```python
from build123d import *

# Parameters (mm, degrees)
BOSS_EXTRUDE1_DEPTH      = 20
SCHIZZO6_R               = 3
TAGLIO_ESTRUSIONE1_DEPTH = 282.870567709


with BuildPart() as part:
    # Sketch1 → Boss-Extrude1 (new body)
    with BuildSketch(Plane.XY):
        Polygon((35, -64), (-43.999999997, -64), (-43.999999997, 126), (35, 126), (251.346408251, 59.694869443), (251.346408251, -64), align=None)
    extrude(amount=BOSS_EXTRUDE1_DEPTH)

    # Schizzo6 → Taglio-Estrusione1 (cut, through all)
    with BuildSketch(Plane.XY.offset(20)):
        with Locations((28.5, -53.5)):
            Circle(SCHIZZO6_R)
        with Locations((-28.5, -53.5)):
            Circle(SCHIZZO6_R)
        with Locations((-28.5, -8.5)):
            Circle(SCHIZZO6_R)
        with Locations((28.5, -8.5)):
            Circle(SCHIZZO6_R)
        with Locations((28.5, 115.5)):
            Circle(SCHIZZO6_R)
        with Locations((28.5, 70.5)):
            Circle(SCHIZZO6_R)
        with Locations((-28.5, 115.5)):
            Circle(SCHIZZO6_R)
        with Locations((-28.5, 70.5)):
            Circle(SCHIZZO6_R)
        with Locations((-38.999999997, 20.3)):
            Circle(SCHIZZO6_R)
        with Locations((-38.999999997, 42.3)):
            Circle(SCHIZZO6_R)
        with Locations((-0.999999997, 20.3)):
            Circle(SCHIZZO6_R)
        with Locations((-0.999999997, 42.3)):
            Circle(SCHIZZO6_R)
    extrude(amount=-TAGLIO_ESTRUSIONE1_DEPTH, mode=Mode.SUBTRACT)


solid = part.part
```
Input: part model. Units: mm. Frame: model coordinates. Round coordinates to 2 decimals unless told otherwise and drop trailing zeros. Order: outer loops, then holes, each group sorted by start corner. A loop starts at its lowest first (then second) coordinate and runs counter-clockwise, first axis right, second up. Notation, with made-up numbers: (80.25, 63) - (89.25, 63) arc R35 ccw to (89.25, 99) - close; hole circle Ø8 at (-18, -14). An arc over 180 degrees is marked (long way). One line per question, with ' | ' between items. Start each with the question number.
1) Contact query for a flat-ended pin moving along its axis: P1, Ø7, axis at x = -1, y = 20.3, coming from the -Z side. Output: stop coordinate, or through.
2) Ray query, probe 1 along Y at (x, z) = (-39, 14); probe 2 along Y at (x, z) = (30.5, 1.25); probe 3 along X at (y, z) = (43, 14.25). Return the intervals inside material, ascending.
3) Cut plane D-D, the plane x = 230. Return the cut outline in (y, z).
4) Cut plane B-B, the plane y = -8.5. Return the cut outline in (x, z).
5) Cut plane A-A, the plane x = -1. Return the cut outline in (y, z), then the cut area to 3 significant figures.
6) Pull-direction query (X, two-part tool) for faces 1 (the cylindrical face through (25.5, -8.4, 10.1)), 2 (the flat face through (-5, 126, 10)), 3 (the flat face through (141.7, 93.3, 9.9)), 4 (the flat face through (-44, 30, 10)); classes: +X half, -X half, draft (parallel to the pull), parting line (faces both ways), or undercut.
7) Cut plane C-C, the plane z = 5. Give the number of separate pieces and of enclosed holes in the cut face, then the cut area to 3 significant figures.
Worked out:
1) P1: stops at z = 0
2) probe 1: y = -64 to 17.3, 23.3 to 39.3, 45.3 to 126 | probe 2: y = -64 to -55.74, -51.26 to -10.74, -6.26 to 68.26, 72.74 to 113.26, 117.74 to 126 | probe 3: x = -44 to -41.92, -36.08 to -3.92, 1.92 to 251.35
3) outline: (-64, 0) - (66.24, 0) - (66.24, 20) - (-64, 20) - close
4) outline: (-44, 0) - (-31.5, 0) - (-31.5, 20) - (-44, 20) - close; (-25.5, 0) - (25.5, 0) - (25.5, 20) - (-25.5, 20) - close; (31.5, 0) - (251.35, 0) - (251.35, 20) - (31.5, 20) - close
5) outline: (-64, 0) - (17.3, 0) - (17.3, 20) - (-64, 20) - close; (23.3, 0) - (39.3, 0) - (39.3, 20) - (23.3, 20) - close; (45.3, 0) - (126, 0) - (126, 20) - (45.3, 20) - close | area: 3,560 mm^2
6) face 1: undercut | face 2: draft | face 3: +X half | face 4: -X half
7) separate pieces: 1 | enclosed holes: 12 | area: 48,600 mm^2
